Here's the drawing with two shaded views (mm, measured from the low corner). I have some questions. A direction names the side the tool comes from. Give positions to 0.01 mm unless a question says otherwise; leave off trailing zeros. Write each loop counter-clockwise with the first axis right and the second up, starting at its lowest first coordinate (ties: lowest second). Pieces come first, ordered by that corner, then holes. Notation, with made-up numbers: M -36,-39 L 3,-39 A24 ccw 3,-9 Z; hole C 69.5,87.5 d5. An arc over 180 degrees is marked long. Use one line per item in the form item = value.
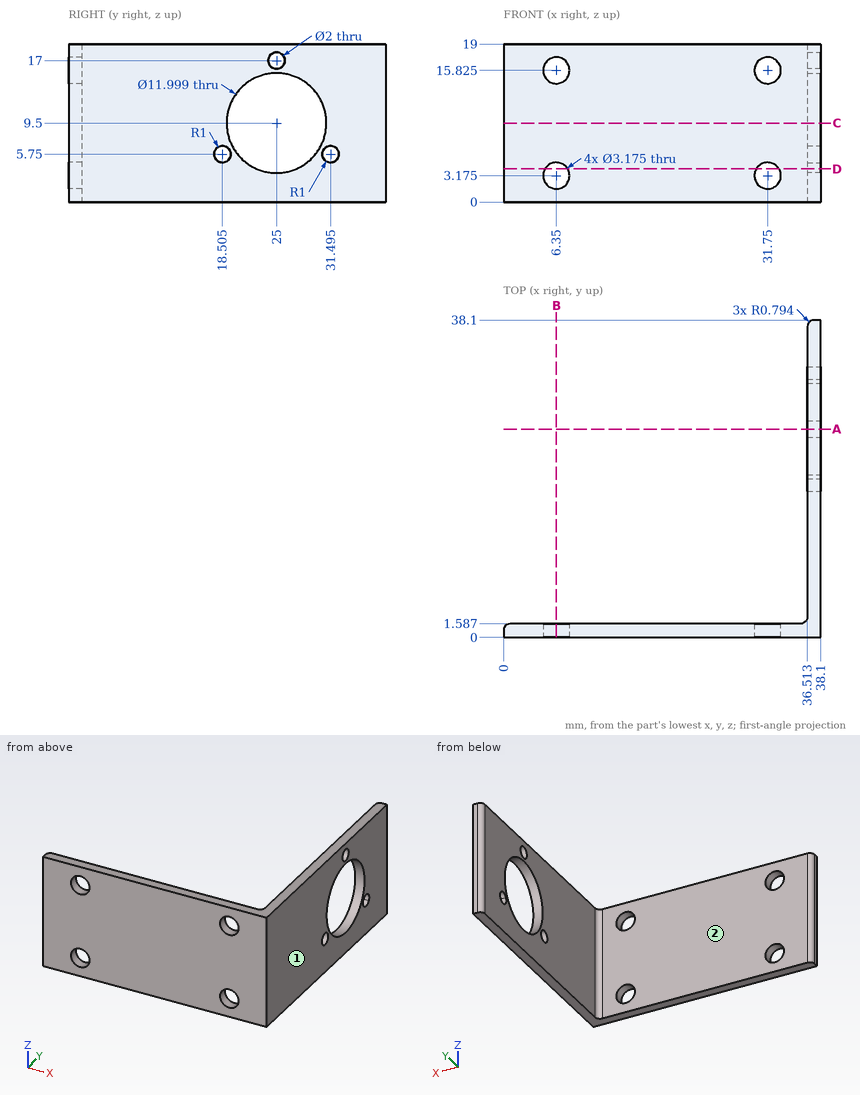
1) I want a section at A-A, the plane y = 25. Please give me the cut outline in (x, z).
Checked values:
outline = M 36.51,0 L 38.1,0 L 38.1,3.5 L 36.51,3.5 Z; M 36.51,15.5 L 38.1,15.5 L 38.1,16 L 36.51,16 Z; M 36.51,18 L 38.1,18 L 38.1,19 L 36.51,19 Z
2) I want a section at D-D, the plane z = 4. Please give me the cut outline in (x, y).
Checked values:
outline = M 0,0 L 4.99,0 L 4.99,1.59 L 0.79,1.59 A0.79 ccw 0,0.79 Z; M 7.71,0 L 30.39,0 L 30.39,1.59 L 7.71,1.59 Z; M 33.11,0 L 38.1,0 L 38.1,22.6 L 36.51,22.6 L 36.51,2.38 A0.79 cw 35.72,1.59 L 33.11,1.59 Z; M 36.51,27.4 L 38.1,27.4 L 38.1,38.1 L 37.31,38.1 A0.79 ccw 36.51,37.31 Z
3) I want a section at C-C, the plane z = 9.5. Please give me the cut outline in (x, y).
Checked values:
outline = M 0,0 L 38.1,0 L 38.1,19 L 36.51,19 L 36.51,2.38 A0.79 cw 35.72,1.59 L 0.79,1.59 A0.79 ccw 0,0.79 Z; M 36.51,31 L 38.1,31 L 38.1,38.1 L 37.31,38.1 A0.79 ccw 36.51,37.31 Z
4) I want a section at B-B, the plane x = 6.35. Please give me the cut outline in (y, z).
Checked values:
outline = M 0,0 L 1.59,0 L 1.59,1.59 L 0,1.59 Z; M 0,4.76 L 1.59,4.76 L 1.59,14.24 L 0,14.24 Z; M 0,17.41 L 1.59,17.41 L 1.59,19 L 0,19 Z
5) For the marked faces 1 and 2, which set-ups out of +Z, -Z, +X, -X, +Y, -Y let a thin tool reach every point of the face, with its end or its side?
Checked values:
face_1 = +Z, -Z, +X, +Y, -Y
face_2 = +Z, -Z, -X, +Y
6) If I drill on L1, parallel to Z at x = 31.75, y = 1.2; L2, parallel to Y at x = 37.6, z = 9.5; L3, parallel to X at y = 17, z = 6, over which ranges is the centre line in solid material (lowest first)?
Checked values:
L1 = 0 to 1.59, 4.76 to 14.24, 17.41 to 19
L2 = 0 to 19, 31 to 38.1
L3 = 36.51 to 38.1
7) For pin 1 Ø3.5 at (x, z) = (6.35, 3.175) entering from +Y; pin 2 Ø1.9 at (x, z) = (31.75, 3.175) entering from +Y; pin 3 Ø2.5 at (y, z) = (25, 17) entering from -X; pin 4 Ø6 at (x, z) = (34, 6) entering from +Y, each with a flat end and sliding along its axis, tell me the tip position at first contact or that it passes through.
Checked values:
pin_1 = 1.59
pin_2 = through
pin_3 = 36.51
pin_4 = 38.04
